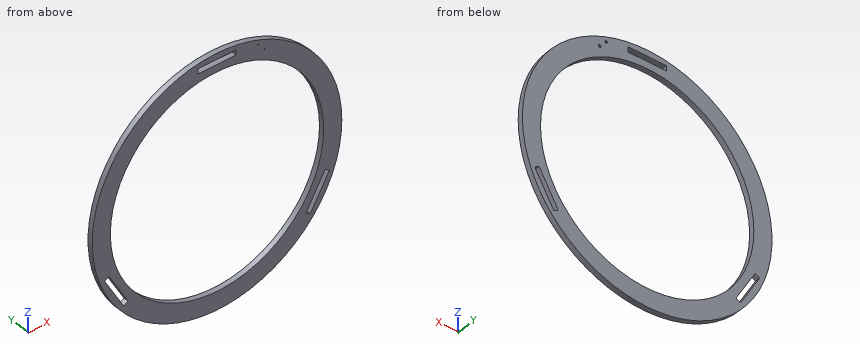
```python
from build123d import *

# Parameters (mm, degrees)
SKETCH1_R                      = 292.5
SKETCH1_R_2                    = 250
BOSS_EXTRUDE1_DEPTH            = 12
SKETCH2_W                      = 90
SKETCH2_H                      = 12
CUT_EXTRUDE1_DEPTH             = 12
CIRPATTERN1_COUNT              = 3
CBORE_FOR_M3_SHCS1_D           = 3.4
CBORE_FOR_M3_SHCS1_CBORE_D     = 6.5
CBORE_FOR_M3_SHCS1_CBORE_DEPTH = 3


with BuildPart() as part:
    # Sketch1 → Boss-Extrude1 (new body)
    with BuildSketch(Plane(origin=(0, 0, 0), x_dir=(1, 0, 0), z_dir=(0, 1, 0))):
        Circle(SKETCH1_R)
        Circle(SKETCH1_R_2, mode=Mode.SUBTRACT)
    extrude(amount=BOSS_EXTRUDE1_DEPTH)

    # Sketch2 → Cut-Extrude1 (cut)
    with BuildSketch(Plane(origin=(0, 12, 0), x_dir=(1, 0, 0), z_dir=(0, 1, 0))):
        with Locations((0, -272.5)):
            Rectangle(SKETCH2_W, SKETCH2_H)
    cut_extrude1 = extrude(amount=-CUT_EXTRUDE1_DEPTH, mode=Mode.SUBTRACT)

    # CirPattern1: Cut-Extrude1 ×3 about axis
    cirpattern1_axis = Axis((0, 0, 0), (0, 1, 0))
    for i in range(1, CIRPATTERN1_COUNT):
        add(cut_extrude1.rotate(cirpattern1_axis, i * 360 / CIRPATTERN1_COUNT), mode=Mode.SUBTRACT)

    # CBORE for M3 SHCS1 (through all)
    with Locations(Plane(origin=(0, 12, 0), x_dir=(1, 0, 0), z_dir=(0, 1, 0))):
        with Locations((111.175516554, -247.940494387), (96.081953174, -265.03974421)):
            CounterBoreHole(CBORE_FOR_M3_SHCS1_D / 2, CBORE_FOR_M3_SHCS1_CBORE_D / 2, CBORE_FOR_M3_SHCS1_CBORE_DEPTH)


solid = part.part
```
Could you check a few things on this model? Use its own coordinates, in mm. Round coordinates to 2 decimals unless told otherwise and drop trailing zeros. Loops run counter-clockwise (first coordinate to the right, second up) from the corner with the lowest first, then second, coordinate; pieces in that order, holes last. Notation, with made-up numbers: (77.5, 59) - (94.5, 59) arc R24 ccw to (94.5, 87) - close; hole circle Ø4 at (73, 74.5). An arc over 180 degrees is marked (long way). Answer as CSV lines item,"result".
1. I want a section at B-B on z = 0. List the corners of the cut face in (x, y) for me.
Filled in:
outline,"(-292.5, 0) - (-250, 0) - (-250, 12) - (-292.5, 12) - close; (250, 0) - (292.5, 0) - (292.5, 12) - (250, 12) - close"
2. Please list where these lines run through material, in increasing order: line 1 along Z through (x, y) = (0, 3.25); line 2 along X through (y, z) = (8.5, -175.5); line 3 along Z through (x, y) = (-230, 7). Write a range as [from, to].
Filled in:
line 1,"z = [-292.5, -250], [250, 266.5], [278.5, 292.5]"
line 2,"x = [-234, -220.26], [-213.97, -178.04], [178.04, 213.97], [220.26, 234]"
line 3,"z = [-180.71, -158.63], [-134.63, -97.98], [97.98, 180.71]"
3. I want a section at C-C on x = -72.5. List the corners of the cut face in (y, z) for me, then the cut area to 3 significant figures.
Filled in:
outline,"(0, -283.37) - (12, -283.37) - (12, -239.26) - (0, -239.26) - close; (0, 239.26) - (12, 239.26) - (12, 283.37) - (0, 283.37) - close"
area,"1,060 mm^2"
4. For pin 1 Ø1 at (x, y) = (230.5, 5.5) entering from -Z; pin 2 Ø4 at (x, z) = (111.18, 247.94) entering from +Y; pin 3 Ø2 at (x, z) = (96.08, 265.04) entering from +Y; pin 4 Ø5 at (x, y) = (160.5, 2) entering from +Z, each with a flat end and sliding along its axis, tell me the tip position at first contact or that it passes through.
Filled in:
pin 1,"stops at z = -180.71"
pin 2,"stops at y = 9"
pin 3,"passes through"
pin 4,"stops at z = 246.15"
5. I want a section at A-A on x = 0. List the corners of the cut face in (y, z) for me.
Filled in:
outline,"(0, -292.5) - (12, -292.5) - (12, -250) - (0, -250) - close; (0, 250) - (12, 250) - (12, 266.5) - (0, 266.5) - close; (0, 278.5) - (12, 278.5) - (12, 292.5) - (0, 292.5) - close"
6. I want a section at D-D on y = 3. List the corners of the cut face in (x, z) for me, then the cut area to 3 significant figures.
Filled in:
outline,"circle Ø585 at (0, 0); hole (-263.69, -100.28) - (-218.69, -178.22) - (-208.3, -172.22) - (-253.3, -94.28) - close; hole circle Ø500 at (0, 0); hole (-45, 266.5) - (45, 266.5) - (45, 278.5) - (-45, 278.5) - close; hole circle Ø3.4 at (96.08, 265.04); hole circle Ø3.4 at (111.18, 247.94); hole (208.3, -172.22) - (218.69, -178.22) - (263.69, -100.28) - (253.3, -94.28) - close"
area,"69,200 mm^2"
